from build123d import *

# Parameters (mm, degrees)
SKETCH_1_R          = 44.5
SKETCH_1_R_2        = 40.5
EXTRUDE_1_DEPTH     = 2
SKETCH_2_R          = 44.5
SKETCH_2_R_2        = 42.1
EXTRUDE_2_DEPTH     = 3.1
SKETCH_3_R          = 51.5
SKETCH_3_R_2        = 42.1
EXTRUDE_3_DEPTH     = 2
SKETCH_6_R          = 1.4
CUT_EXTRUDE_3_DEPTH = 74.177250563
CHAMFER_1_SIZE      = 0.5
CHAMFER_2_SIZE      = 0.5


with BuildPart() as part:
    # 스케치1 → 보스-돌출1 (new body)
    with BuildSketch(Plane(origin=(0, 0, 0), x_dir=(1, 0, 0), z_dir=(0, 1, 0))):
        with Locations(Location((0, 0, 0), (0, 0, 270))):
            Circle(SKETCH_1_R)
        with Locations(Location((0, 0, 0), (0, 0, 270))):
            Circle(SKETCH_1_R_2, mode=Mode.SUBTRACT)
    extrude(amount=EXTRUDE_1_DEPTH)

    # 스케치2 → 보스-돌출2 (add)
    with BuildSketch(Plane(origin=(0, 2, 0), x_dir=(1, 0, 0), z_dir=(0, 1, 0))):
        with Locations(Location((0, 0, 0), (0, 0, 270))):
            Circle(SKETCH_2_R)
        with Locations(Location((0, 0, 0), (0, 0, 90))):
            Circle(SKETCH_2_R_2, mode=Mode.SUBTRACT)
    extrude(amount=EXTRUDE_2_DEPTH)

    # 스케치3 → 보스-돌출3 (add)
    with BuildSketch(Plane(origin=(0, 5.1, 0), x_dir=(1, 0, 0), z_dir=(0, 1, 0))):
        with Locations(Location((0, 0, 0), (0, 0, 270))):
            Circle(SKETCH_3_R)
        with Locations(Location((0, 0, 0), (0, 0, 90))):
            Circle(SKETCH_3_R_2, mode=Mode.SUBTRACT)
    extrude(amount=EXTRUDE_3_DEPTH)

    # 스케치6 → 컷-돌출3 (cut, through all)
    with BuildSketch(Plane(origin=(0, 7.1, 0), x_dir=(1, 0, 0), z_dir=(0, 1, 0))):
        with Locations(Location((0, 47.1, 0), (0, 0, 270))):
            Circle(SKETCH_6_R)
        with Locations(Location((27.684685383, 38.104700435, 0), (0, 0, 270))):
            Circle(SKETCH_6_R)
        with Locations(Location((44.794761918, 14.554700435, 0), (0, 0, 270))):
            Circle(SKETCH_6_R)
        with Locations(Location((44.794761918, -14.554700435, 0), (0, 0, 270))):
            Circle(SKETCH_6_R)
        with Locations(Location((27.684685383, -38.104700435, 0), (0, 0, 270))):
            Circle(SKETCH_6_R)
        with Locations(Location((0, -47.1, 0), (0, 0, 270))):
            Circle(SKETCH_6_R)
        with Locations(Location((-27.684685383, -38.104700435, 0), (0, 0, 270))):
            Circle(SKETCH_6_R)
        with Locations(Location((-44.794761918, -14.554700435, 0), (0, 0, 270))):
            Circle(SKETCH_6_R)
        with Locations(Location((-44.794761918, 14.554700435, 0), (0, 0, 270))):
            Circle(SKETCH_6_R)
        with Locations(Location((-27.684685383, 38.104700435, 0), (0, 0, 270))):
            Circle(SKETCH_6_R)
    extrude(amount=-CUT_EXTRUDE_3_DEPTH, mode=Mode.SUBTRACT)

    # 모따기1
    chamfer_1_edges = [part.edges().sort_by_distance(p)[0] for p in [
        (0, 5.1, -48.5),
        (-27.684685383, 5.1, -39.504700435),
        (-44.794761918, 5.1, -15.954700435),
        (-44.794761918, 5.1, 13.154700435),
        (-27.684685383, 5.1, 36.704700435),
        (0, 5.1, 45.7),
        (27.684685383, 5.1, 36.704700435),
        (44.794761918, 5.1, 13.154700435),
        (44.794761918, 5.1, -15.954700435),
        (27.684685383, 5.1, -39.504700435),
    ]]
    chamfer(chamfer_1_edges, length=CHAMFER_1_SIZE)

    # 모따기2
    chamfer_2_edges = [part.edges().sort_by_distance(p)[0] for p in [
        (0, 5.1, -44.5),
        (0, 7.1, 42.1),
    ]]
    chamfer(chamfer_2_edges, length=CHAMFER_2_SIZE)


solid = part.part
CAD build for the part. Positions are in the model's coordinates, mm. A direction names the side the tool comes from. Coordinates: 2 decimals unless noted, no trailing zeros. Order: outer loops, then holes, each group sorted by start corner. A loop starts at its lowest first (then second) coordinate and runs counter-clockwise, first axis right, second up.
Item 1: Band-saw the part on D-D on z = -47.1. List the corners of the cut face in (x, y).
Check sheet entries:
outline: (-20.83, 5.1) - (-1.9, 5.1) - (-1.4, 5.6) - (-1.4, 7.1) - (-20.83, 7.1) - close; (1.4, 5.6) - (1.9, 5.1) - (20.83, 5.1) - (20.83, 7.1) - (1.4, 7.1) - close
Item 2: 3-axis set-ups, long thin cutter, end or side, ignore diameter. For faces 1 (the face through (22, 2, -35)), 2 (the face through (-45.69, 6.09, 23.76)): which of +Z, -Z, +X, -X, +Y, -Y reach the whole face in a straight line?
Check sheet entries:
face 1: +Y
face 2: +Y, -Y
Item 3: Band-saw the part on A-A on z = 0. List the corners of the cut face in (x, y).
Check sheet entries:
outline: (-51.5, 5.1) - (-45, 5.1) - (-44.5, 4.6) - (-44.5, 0) - (-40.5, 0) - (-40.5, 2) - (-42.1, 2) - (-42.1, 6.6) - (-42.6, 7.1) - (-51.5, 7.1) - close; (40.5, 0) - (44.5, 0) - (44.5, 4.6) - (45, 5.1) - (51.5, 5.1) - (51.5, 7.1) - (42.6, 7.1) - (42.1, 6.6) - (42.1, 2) - (40.5, 2) - close
Item 4: Pin check, flat tips, straight feed: pin 1 Ø4.5 at (x, z) = (27.68, 38.1) entering from -Y; pin 2 Ø1 at (x, y) = (-15, 6.5) entering from +Z; pin 3 Ø3 at (x, z) = (-44.79, 14.55) entering from -Y. Stop position of each tip, or through.
Check sheet entries:
pin 1: stops at y = 4.94
pin 2: stops at z = 49.42
pin 3: stops at y = 5.49
Item 5: Two-plate mould, pull along X, no slides. Class faces 3 (the face through (30.075, 2.268, -32.798)), 4 (the face through (38.4, 7.1, -19.3)), 5 (the face through (0.421, 6.36, 48.435)): +X half, -X half, draft (parallel to the pull), parting line (faces both ways), or undercut.
Check sheet entries:
face 3: parting line
face 4: draft
face 5: undercut
Item 6: Band-saw the part on B-B on x = 0. Give the number of separate pieces and of enclosed holes in the cut face, plus the area to 3 significant figures.
Check sheet entries:
separate pieces: 4
enclosed holes: 0
area: 56.8 mm2
Item 7: Drill centre lines: L1, parallel to Y at x = -8.5, z = 40.5; L2, parallel to X at y = 1, z = -5; L3, parallel to Z at x = -11, y = 1.25. Where is each one in solid material? Low to high.
Check sheet entries:
L1: y = 0 to 2
L2: x = -44.22 to -40.19, 40.19 to 44.22
L3: z = -43.12 to -38.98, 38.98 to 43.12
